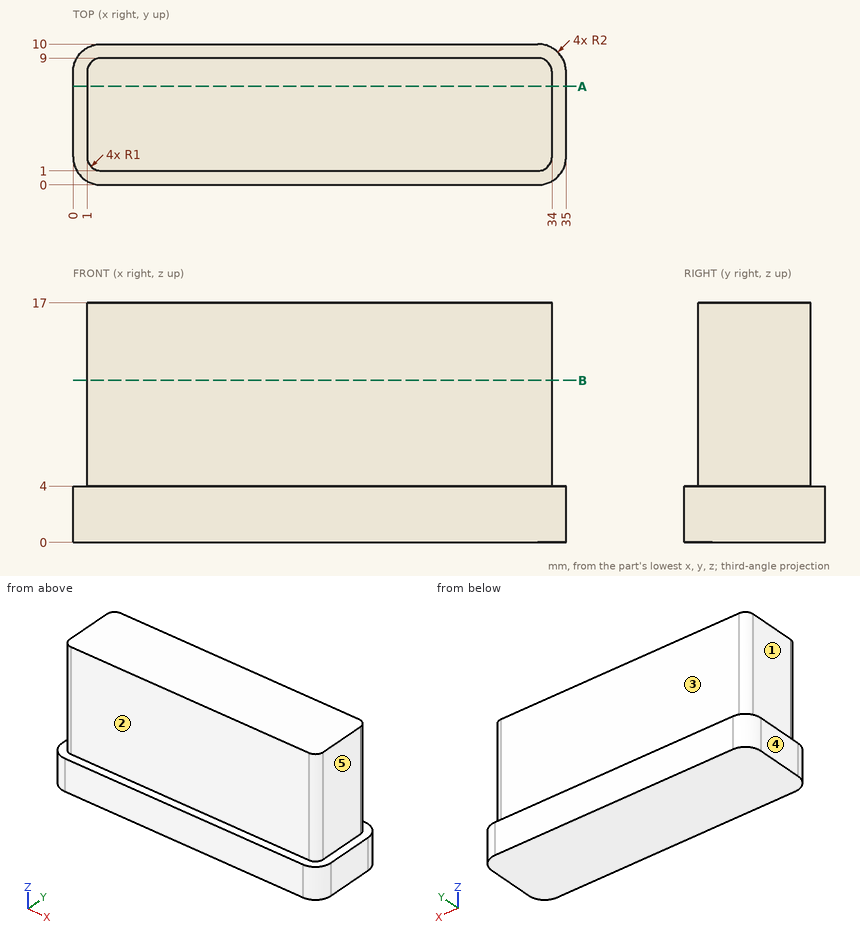
Can you work these out from the drawing? Everything is in mm from the part's minimum corner. A direction names the side the tool comes from. Give positions to 0.01 mm unless a question says otherwise; leave off trailing zeros. Write each loop counter-clockwise with the first axis right and the second up, starting at its lowest first coordinate (ties: lowest second). Pieces come first, ordered by that corner, then holes. Notation, with made-up numbers: (-14.75, 38.5) -> (34.25, 38.5) arc R29 cw to (34.25, 64.5) -> close; hole circle Ø5 at (14, -25). An arc over 180 degrees is marked (long way). Write each question's results on one line, items separated by ' | '.
Item 1: Suppose I cut it at A-A on y = 7. Write out the boundary of the cut face in (x, z), plus the area to 3 significant figures.
Output:
outline: (0, 0) -> (35, 0) -> (35, 4) -> (34, 4) -> (34, 17) -> (1, 17) -> (1, 4) -> (0, 4) -> close | area: 569 mm^2
Item 2: If I drill on L1, parallel to Y at x = 23, z = 10; L2, parallel to X at y = 2.25, z = 15; L3, parallel to Z at x = 15.5, y = 0.5, over which ranges is the centre line in solid material (lowest first)?
Output:
L1: y = 1 to 9 | L2: x = 1 to 34 | L3: z = 0 to 4
Item 3: Suppose I cut it at B-B on z = 11.5. Write out the boundary of the cut face in (x, y).
Output:
outline: (1, 2) arc R1 ccw to (2, 1) -> (33, 1) arc R1 ccw to (34, 2) -> (34, 8) arc R1 ccw to (33, 9) -> (2, 9) arc R1 ccw to (1, 8) -> close
Item 4: For pin 1 Ø5 at (y, z) = (5.5, 10.5) entering from -X; pin 2 Ø5 at (x, y) = (5, 5) entering from -Z; pin 3 Ø1 at (x, z) = (31, 12.5) entering from +Y; pin 4 Ø8 at (x, z) = (21.5, 10.5) entering from -Y, each with a flat end and sliding along its axis, tell me the tip position at first contact or that it passes through.
Output:
pin 1: stops at x = 1 | pin 2: stops at z = 0 | pin 3: stops at y = 9 | pin 4: stops at y = 1
Item 5: On a 3-axis mill with a long thin cutter (end or side, diameter ignored), from which of +Z, -Z, +X, -X, +Y, -Y can I reach the whole of each face in a straight line? I mean the marked faces 1, 2, 3, 4 and 5. Say none if no direction works.
Output:
face 1: +Z, -X, +Y, -Y | face 2: +Z, +X, -X, -Y | face 3: +Z, +X, -X, +Y | face 4: +Z, -Z, -X, +Y, -Y | face 5: +Z, +X, +Y, -Y
